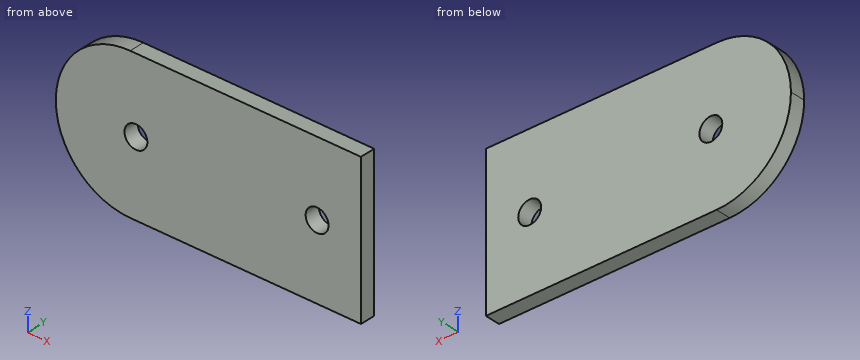
```python
from build123d import *

# Parameters (mm, degrees)
SKETCH1_W           = 40
SKETCH1_H           = 19.5
SKETCH1_R           = 1.5
BOSS_EXTRUDE1_DEPTH = 2
FILLET1_R           = 9.75


with BuildPart() as part:
    # Sketch1 → Boss-Extrude1 (new body)
    with BuildSketch(Plane(origin=(0, 0, 0), x_dir=(1, 0, 0), z_dir=(0, 1, 0))):
        Rectangle(SKETCH1_W, SKETCH1_H)
        with Locations(Location((-9.5, 0, 0), (0, 0, 270))):
            Circle(SKETCH1_R, mode=Mode.SUBTRACT)
        with Locations(Location((14.25, 0, 0), (0, 0, 270))):
            Circle(SKETCH1_R, mode=Mode.SUBTRACT)
    extrude(amount=BOSS_EXTRUDE1_DEPTH)

    # Fillet1
    fillet1_edges = [part.edges().sort_by_distance(p)[0] for p in [
        (-20, 1, -9.75),
        (-20, 1, 9.75),
    ]]
    fillet(fillet1_edges, radius=FILLET1_R - 0.0001)  # a hair under: the kernel refuses the full size


solid = part.part
```
CAD build for the part. Positions are in the model's coordinates, mm. Round coordinates to 2 decimals unless told otherwise and drop trailing zeros. Order: outer loops, then holes, each group sorted by start corner. A loop starts at its lowest first (then second) coordinate and runs counter-clockwise, first axis right, second up.
Q1. Slice it at D-D (z = 8). Write the cut outline in (x, y).
Q2. Slice it at A-A (x = 14.25). Write the cut outline in (y, z), and give its area (3 significant figures).
Q3. Slice it at C-C (z = -3.75). Write the cut outline in (x, y), and give its area (3 significant figures).
Q4. Slice it at B-B (y = 0.4). State how many separate pieces and enclosed holes the cut face has, and give its area (3 significant figures).
Q5. Wall check: L1, parallel to X at y = 0.6, z = 0; L2, parallel to Z at x = 15, y = 1.85; L3, parallel to Z at x = -9, y = 0.45. Give the ranges that are in metal, low to high.
Q6. Drop a flat-ended pin along its axis: pin 1 (4 mm diameter, centred on x = -12, z = 2.5, fed in from -Y). Give the stop position or say it passes through.
Results below:
1. outline: (-15.82, 0) - (20, 0) - (20, 2) - (-15.82, 2) - close
2. outline: (0, -9.75) - (2, -9.75) - (2, -1.5) - (0, -1.5) - close; (0, 1.5) - (2, 1.5) - (2, 9.75) - (0, 9.75) - close
2. area: 33.0 mm2
3. outline: (-19.25, 0) - (20, 0) - (20, 2) - (-19.25, 2) - close
3. area: 78.5 mm2
4. separate pieces: 1
4. enclosed holes: 2
4. area: 725 mm2
5. L1: x = -20 to -11, -8 to 12.75, 15.75 to 20
5. L2: z = -9.75 to -1.3, 1.3 to 9.75
5. L3: z = -9.75 to -1.41, 1.41 to 9.75
6. pin 1: stops at y = 0
